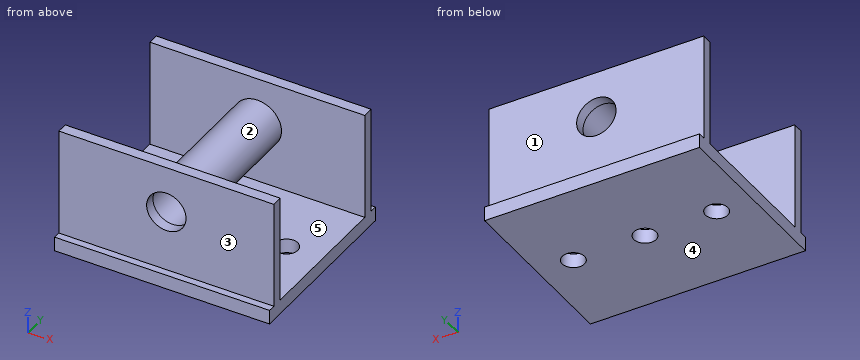
from build123d import *

# Parameters (mm, degrees)
SKETCH_1_W          = 120
SKETCH_1_H          = 100
SKETCH_1_R          = 6.25
EXTRUDE_1_DEPTH     = 8
SKETCH_2_W          = 120
SKETCH_2_H          = 6
EXTRUDE_2_DEPTH     = 60
SKETCH_3_R          = 11
CUT_EXTRUDE_1_DEPTH = 133.060592154
EXTRUDE_3_REACH     = 129.765
SKETCH_4_R          = 13.5
SKETCH_4_R_2        = 11


with BuildPart() as part:
    # Эскиз1 → Бобышка-Вытянуть1 (new body)
    with BuildSketch(Plane.XY):
        Rectangle(SKETCH_1_W, SKETCH_1_H)
        Circle(SKETCH_1_R, mode=Mode.SUBTRACT)
        with Locations((40, 0)):
            Circle(SKETCH_1_R, mode=Mode.SUBTRACT)
        with Locations(Location((-40, 0, 0), (0, 0, 180))):
            Circle(SKETCH_1_R, mode=Mode.SUBTRACT)
    extrude(amount=EXTRUDE_1_DEPTH)

    # Эскиз2 → Бобышка-Вытянуть2 (add)
    with BuildSketch(Plane.XY.offset(8)):
        with Locations((0, -43)):
            Rectangle(SKETCH_2_W, SKETCH_2_H)
        with Locations((0, 43)):
            Rectangle(SKETCH_2_W, SKETCH_2_H)
    extrude(amount=EXTRUDE_2_DEPTH)

    # Эскиз3 → Вырез-Вытянуть1 (cut, through all)
    with BuildSketch(Plane.XZ.offset(46)):
        with Locations(Location((0, 42, 0), (0, 0, 270))):
            Circle(SKETCH_3_R)
    extrude(amount=-CUT_EXTRUDE_1_DEPTH, mode=Mode.SUBTRACT)

    # Эскиз4 → Бобышка-Вытянуть3 (add, up to next)
    with BuildSketch(Plane.XZ.offset(-40), mode=Mode.PRIVATE) as extrude_3_sk1:
        with Locations(Location((0, 42, 0), (0, 0, 90))):
            Circle(SKETCH_4_R)
        with Locations(Location((0, 42, 0), (0, 0, 270))):
            Circle(SKETCH_4_R_2, mode=Mode.SUBTRACT)
    extrude_3_tool1 = extrude(extrude_3_sk1.sketch, amount=EXTRUDE_3_REACH, mode=Mode.PRIVATE) - part.part
    add(extrude_3_tool1.solids().sort_by_distance((0, 40, 28.881838))[0])


solid = part.part
Verification items for the finished model (mm, model axes). Face numbers are marked on the shaded views. A direction names the side the tool comes from. Give positions to 0.01 mm unless a question says otherwise; leave off trailing zeros. Write each loop counter-clockwise with the first axis right and the second up, starting at its lowest first coordinate (ties: lowest second). Pieces come first, ordered by that corner, then holes.
(1) Mould release check, pull along Z, two halves, no side actions. Record for the marked faces 3, 4 and 5: +Z half, -Z half, draft (parallel to the pull), parting line (faces both ways), or undercut.
(2) Gauge pin test, flat ends, axial feed: pin 1 (1.2 mm diameter, centred on x = -9.5, y = -47.5, fed in from +Z); pin 2 (12 mm diameter, centred on x = 33, z = 52, fed in from +Y); pin 3 (1.5 mm diameter, centred on x = -14, z = 52.5, fed in from -Y); pin 4 (1 mm diameter, centred on x = 41.5, y = -15, fed in from -Z). Record the tip position at first contact, or that the pin passes through.
(3) Cross-section at B-B (z = 19.5). Enter the section's corners in (x, y), plus the area to 3 significant figures.
(4) Access from +Z, -Z, +X, -X, +Y, -Y to the whole of each face (thin tool, end or side, straight path). Record for the marked faces 1 and 2.
(5) Cross-section at D-D (y = -31). Enter the section's corners in (x, z).
(6) Cross-section at C-C (x = 0). Enter the section's corners in (y, z).
(7) Material ranges on line 1 (Y direction, x = 0, z = 5); line 2 (Y direction, x = -1, z = 62.5); line 3 (X direction, y = 11, z = 42), recorded low to high.
(8) Cross-section at A-A (y = 0). Enter the section's corners in (x, z).
Worked out:
1. face 3: draft
1. face 4: -Z half
1. face 5: undercut
2. pin 1: stops at z = 8
2. pin 2: stops at y = 46
2. pin 3: stops at y = -46
2. pin 4: stops at z = 0
3. outline: (-60, -46) - (60, -46) - (60, -40) - (-60, -40) - close; (-60, 40) - (60, 40) - (60, 46) - (-60, 46) - close
3. area: 1,440 mm2
4. face 1: +Z, +X, -X, +Y
4. face 2: none
5. outline: (-60, 0) - (60, 0) - (60, 8) - (-60, 8) - close; circle Ø27 at (0, 42); hole circle Ø22 at (0, 42)
6. outline: (-50, 0) - (-6.25, 0) - (-6.25, 8) - (-40, 8) - (-40, 28.5) - (40, 28.5) - (40, 8) - (6.25, 8) - (6.25, 0) - (50, 0) - (50, 8) - (46, 8) - (46, 31) - (-46, 31) - (-46, 8) - (-50, 8) - close; (-46, 53) - (46, 53) - (46, 68) - (40, 68) - (40, 55.5) - (-40, 55.5) - (-40, 68) - (-46, 68) - close
7. line 1: y = -50 to -6.25, 6.25 to 50
7. line 2: y = -46 to -40, 40 to 46
7. line 3: x = -13.5 to -11, 11 to 13.5
8. outline: (-60, 0) - (-46.25, 0) - (-46.25, 8) - (-60, 8) - close; (-33.75, 0) - (-6.25, 0) - (-6.25, 8) - (-33.75, 8) - close; circle Ø27 at (0, 42); (6.25, 0) - (33.75, 0) - (33.75, 8) - (6.25, 8) - close; (46.25, 0) - (60, 0) - (60, 8) - (46.25, 8) - close; hole circle Ø22 at (0, 42)
